```python
from build123d import *

# Parameters (mm, degrees)
F0_W     = 93.043737
F0_H     = 76.870489
F0_R     = 6.35
F1_DEPTH = 71.87439
F2_R     = 10.16
F3_R     = 5.08


with BuildPart() as f1:
    # F0 (on Front) → F1 (new body)
    with BuildSketch(Plane.XZ):
        with Locations((3.710334, -1.617325)):
            Rectangle(F0_W, F0_H)
        with Locations((-30.111535, 24.117919)):
            Circle(F0_R, mode=Mode.SUBTRACT)
        with Locations((-4.711535, 24.117919)):
            Circle(F0_R, mode=Mode.SUBTRACT)
        with Locations((20.688465, 24.117919)):
            Circle(F0_R, mode=Mode.SUBTRACT)
    extrude(amount=F1_DEPTH)

    # F2
    f2_edges = [f1.edges().sort_by_distance(p)[0] for p in [
        (50.232202, -35.937195, 36.817919),
    ]]
    fillet(f2_edges, radius=F2_R)

    # F3
    f3_edges = [f1.edges().sort_by_distance(p)[0] for p in [
        (-1.369667, -71.87439, 36.817919),
    ]]
    fillet(f3_edges, radius=F3_R)


solid = f1.part
```
Work out the finished part from the listing and answer in its coordinate system (mm). Coordinates: 2 decimals unless noted, no trailing zeros. Loops run counter-clockwise (first coordinate to the right, second up) from the corner with the lowest first, then second, coordinate; pieces in that order, holes last.
1) A flat-ended cylindrical pin translates along its axis: pin 1 (11.5 mm diameter, centred on x = -4.71, z = 24.12, fed in from -Y) (3 decimals). Find the tip coordinate at first contact, or state that the pin passes through.
Results:
pin 1: passes through
2) For a pull along X with two mould halves and no side action, classify faces 1 (the flat face through (1, -71.874, -4)), 2 (the cylindrical face through (48.78, -70.35, -7.16)), 3 (the cylindrical face through (23.619, -35.434, 18.484)) as +X half, -X half, draft (parallel to the pull), parting line (faces both ways), or undercut.
Results:
face 1: draft
face 2: +X half
face 3: undercut
3) Section A-A (x = 25) is taken. Give the vertices of the cut face in (y, z), plus the area to 3 significant figures.
Results:
outline: (-71.87, -40.05) - (0, -40.05) - (0, 19.46) - (-71.87, 19.46) - close; (-71.87, 28.78) - (0, 28.78) - (0, 36.82) - (-66.79, 36.82) arc R5.08 ccw to (-71.87, 31.74) - close
area: 4,850 mm2
4) Section B-B (y = -29.5) is taken. Give the vertices of the cut face in (x, z).
Results:
outline: (-42.81, -40.05) - (50.23, -40.05) - (50.23, 26.66) arc R10.16 ccw to (40.07, 36.82) - (-42.81, 36.82) - close; hole circle Ø12.7 at (-30.11, 24.12); hole circle Ø12.7 at (-4.71, 24.12); hole circle Ø12.7 at (20.69, 24.12)
5) Consider probe 1 along X at (y, z) = (-55, 24.5); probe 2 along X at (y, z) = (-63, 29.5); probe 3 along Z at (x, y) = (-7.5, -41). Determine where each line is inside the solid, lowest interval first.
Results:
probe 1: x = -42.81 to -36.45, -23.77 to -11.05, 1.63 to 14.35, 27.03 to 50.23
probe 2: x = -42.81 to -33.48, -26.74 to -8.08, -1.34 to 17.32, 24.06 to 49.83
probe 3: z = -40.05 to 18.41, 29.82 to 36.82
6) Section C-C (x = -6) is taken. Give the vertices of the cut face in (y, z).
Results:
outline: (-71.87, -40.05) - (0, -40.05) - (0, 17.9) - (-71.87, 17.9) - close; (-71.87, 30.34) - (0, 30.34) - (0, 36.82) - (-66.79, 36.82) arc R5.08 ccw to (-71.87, 31.74) - close
